from build123d import *

# Parameters (mm, degrees)
SKETCH1_W           = 200
SKETCH1_H           = 80
BOSS_EXTRUDE1_DEPTH = 3
SKETCH2_R           = 2
CUT_EXTRUDE1_DEPTH  = 108.745069493
FILLET1_R           = 10
SKETCH3_R           = 1.5621
CUT_EXTRUDE2_DEPTH  = 108.745069493
SKETCH4_W           = 20
SKETCH4_H           = 20
CUT_EXTRUDE3_DEPTH  = 108.745069493
FILLET2_R           = 5
CUT_EXTRUDE4_DEPTH  = 108.745069493
SKETCH6_W           = 11.45
SKETCH6_H           = 17.2
CUT_EXTRUDE5_DEPTH  = 108.745069493


with BuildPart() as part:
    # Sketch1 → Boss-Extrude1 (new body)
    with BuildSketch(Plane.XY):
        Rectangle(SKETCH1_W, SKETCH1_H)
    extrude(amount=BOSS_EXTRUDE1_DEPTH)

    # Sketch2 → Cut-Extrude1 (cut, through all)
    with BuildSketch(Plane.XY.offset(3)):
        with Locations((-92, 32)):
            Circle(SKETCH2_R)
        with Locations(Location((-92, -32, 0), (0, 0, 180))):
            Circle(SKETCH2_R)
        with Locations((92, -32)):
            Circle(SKETCH2_R)
        with Locations(Location((92, 32, 0), (0, 0, 180))):
            Circle(SKETCH2_R)
    extrude(amount=-CUT_EXTRUDE1_DEPTH, mode=Mode.SUBTRACT)

    # Fillet1
    fillet1_edges = [part.edges().sort_by_distance(p)[0] for p in [
        (100, -40, 1.5),
        (-100, -40, 1.5),
        (-100, 40, 1.5),
        (100, 40, 1.5),
    ]]
    fillet(fillet1_edges, radius=FILLET1_R)

    # Sketch3 → Cut-Extrude2 (cut, through all)
    with BuildSketch(Plane.XY.offset(3)):
        with Locations((36.6776, 24.1681)):
            Circle(SKETCH3_R)
        with Locations((36.6776, -24.1681)):
            Circle(SKETCH3_R)
        with Locations((-38.4556, -24.1681)):
            Circle(SKETCH3_R)
        with Locations((-45.9486, 24.1681)):
            Circle(SKETCH3_R)
        with Locations((-14.9479, 19.289607234)):
            Circle(SKETCH3_R)
    extrude(amount=-CUT_EXTRUDE2_DEPTH, mode=Mode.SUBTRACT)

    # Sketch4 → Cut-Extrude3 (cut, through all)
    with BuildSketch(Plane.XY.offset(3)):
        with Locations((80, -10)):
            Rectangle(SKETCH4_W, SKETCH4_H)
    extrude(amount=-CUT_EXTRUDE3_DEPTH, mode=Mode.SUBTRACT)

    # Fillet2
    fillet2_edges = [part.edges().sort_by_distance(p)[0] for p in [
        (90, 0, 1.5),
        (90, -20, 1.5),
        (70, -20, 1.5),
        (70, 0, 1.5),
    ]]
    fillet(fillet2_edges, radius=FILLET2_R)

    # Sketch5 → Cut-Extrude4 (cut, through all)
    with BuildSketch(Plane.XY.offset(3)):
        with BuildLine():
            Line((-15, -30), (15, -30))
            ThreePointArc((15, -30), (18, -33), (15, -36))
            Line((15, -36), (-15, -36))
            ThreePointArc((-15, -36), (-18, -33), (-15, -30))
        make_face()
        with BuildLine():
            Line((-15, 30), (15, 30))
            ThreePointArc((15, 30), (18, 33), (15, 36))
            Line((15, 36), (-15, 36))
            ThreePointArc((-15, 36), (-18, 33), (-15, 30))
        make_face()
    extrude(amount=-CUT_EXTRUDE4_DEPTH, mode=Mode.SUBTRACT)

    # Sketch6 → Cut-Extrude5 (cut, through all)
    with BuildSketch(Plane.XY.offset(3)):
        with Locations((80, 19.35)):
            Rectangle(SKETCH6_W, SKETCH6_H)
    extrude(amount=-CUT_EXTRUDE5_DEPTH, mode=Mode.SUBTRACT)


solid = part.part
Check sheet for the modelled part. Datum: model origin and axes. Units: mm. A direction names the side the tool comes from. Round coordinates to 2 decimals unless told otherwise and drop trailing zeros. Write each loop counter-clockwise with the first axis right and the second up, starting at its lowest first coordinate (ties: lowest second). Pieces come first, ordered by that corner, then holes. Notation, with made-up numbers: (-27.5, 89.5) -> (3.5, 89.5) arc R18 cw to (3.5, 98.5) -> close; hole circle Ø2 at (22, -39). An arc over 180 degrees is marked (long way). Answer as CSV lines item,"result". Start each with the question number.
1) Section check C-C on y = 32. Enter the section's corners in (x, z), and give its area (3 significant figures).
2) Release check for a two-part mould opening along Y. For faces 3 (the cylindrical face through (96.99, 37.15, 1.52)), 4 (the cylindrical face through (96.99, -37.15, 1.52)), 5 (the flat face through (-1, 1, 0)), 6 (the cylindrical face through (91.077, 33.774, 1.521)) record: pulls with the +Y half, pulls with the -Y half, needs draft (parallel to the pull), parting line crosses it, or undercut.
3) Section check A-A on y = -18. Enter the section's corners in (x, z).
4) Material ranges on line 1 (Y direction, x = 85, z = 2.05); line 2 (X direction, y = 14, z = 0.25) (3 decimals); line 3 (Y direction, x = -92, z = 1.4), recorded low to high. Write a range as from..to.
5) Go/stop test with flat-tipped pins: P1, Ø12, axis at x = -40.5, y = 4, coming from the -Z side; P2, Ø3, axis at x = 36.68, y = 24.17, coming from the +Z side. Record where each tip stops, or that it passes through.
6) Section check B-B on x = 81. Enter the section's corners in (y, z).
7) Tool access check on faces 1 (the cylindrical face through (72, -1, 1)), 2 (the cylindrical face through (-97.15, -36.99, 1.52)). Record the directions out of +Z, -Z, +X, -X, +Y, -Y that give a thin tool (end or side, any length) a straight path to the whole face; none if there is none.
8) Section check D-D on z = 2.5. State how many separate pieces and enclosed holes the cut face has, and give its area (3 significant figures).
Found:
1,outline,"(-99.8, 0) -> (-94, 0) -> (-94, 3) -> (-99.8, 3) -> close; (-90, 0) -> (-17.83, 0) -> (-17.83, 3) -> (-90, 3) -> close; (17.83, 0) -> (90, 0) -> (90, 3) -> (17.83, 3) -> close; (94, 0) -> (99.8, 0) -> (99.8, 3) -> (94, 3) -> close"
1,area,"468 mm^2"
2,face 3,"pulls with the +Y half"
2,face 4,"pulls with the -Y half"
2,face 5,"needs draft"
2,face 6,"undercut"
3,outline,"(-100, 0) -> (71, 0) -> (71, 3) -> (-100, 3) -> close; (89, 0) -> (100, 0) -> (100, 3) -> (89, 3) -> close"
4,line 1,"y = -40..-20, 0..10.75, 27.95..40"
4,line 2,"x = -100..74.275, 85.725..100"
4,line 3,"y = -39.8..-34, -30..30, 34..39.8"
5,P1,"stops at z = 0"
5,P2,"passes through"
6,outline,"(-40, 0) -> (-20, 0) -> (-20, 3) -> (-40, 3) -> close; (0, 0) -> (10.75, 0) -> (10.75, 3) -> (0, 3) -> close; (27.95, 0) -> (40, 0) -> (40, 3) -> (27.95, 3) -> close"
7,face 1,"+Z, -Z"
7,face 2,"+Z, -Z, -X, -Y"
8,separate pieces,"1"
8,enclosed holes,"13"
8,area,"14,800 mm^2"
